Input: part model. Units: mm. Frame: model coordinates. A direction names the side the tool comes from. Round coordinates to 2 decimals unless told otherwise and drop trailing zeros. Write each loop counter-clockwise with the first axis right and the second up, starting at its lowest first coordinate (ties: lowest second). Pieces come first, ordered by that corner, then holes. Notation, with made-up numbers: (-21.5, 14.25) - (-10.5, 14.25) arc R32 ccw to (-10.5, 48.25) - close; hole circle Ø10 at (-5, 17.5). An arc over 180 degrees is marked (long way). Use one line per item in the form item = value.
Autodesk Inventor part; units mm, degrees
ref_plane "YZ Plane" through (0, 0, 0) normal (1, 0, 0) x (0, 1, 0)
ref_plane "XZ Plane" through (0, 0, 0) normal (0, 1, 0) x (-1, 0, 0)
ref_plane "XY Plane" through (0, 0, 0) normal (0, 0, 1) x (1, 0, 0)
sketch "Sketch1" plane through (0, 0, 0) normal (0, 0, 1) x (1, 0, 0)
  circle A0 centre (0, 0) radius 6
  dimension "d0" = 12
extrude "Extrusion1" add sketch "Sketch1" along normal blind 15
sketch "Sketch2" plane through (0, 0, 0) normal (0, 0, -1) x (-1, 0, 0)
  circle A0 centre (0, 0) radius 6
  circle A1 centre (0, 0) radius 4.699
  dimension "d3" = 9.398
extrude "Extrusion2" cut sketch "Sketch2" against normal blind 7 contours A1
sketch "Sketch3" plane through (0, 0, 15) normal (0, 0, 1) x (1, 0, 0)
  circle A0 centre (0, 0) radius 6
  circle A1 centre (0, 0) radius 3
  dimension "d6" = 6
extrude "Extrusion3" cut sketch "Sketch3" against normal blind 2.5 contours A1
sketch "Sketch4" plane through (0, 0, 15) normal (0, 0, 1) x (1, 0, 0)
  circle A0 centre (0, 0) radius 3
  circle A1 centre (0, 0) radius 6
extrude "Extrusion4" add sketch "Sketch4" along normal blind 15
sketch "Sketch5" plane through (0, 0, 12.5) normal (0, 0, 1) x (1, 0, 0)
  circle A0 centre (0, 0) radius 3
extrude "Extrusion5" add sketch "Sketch5" along normal blind 15
sketch "Sketch6" plane through (0, 0, 30) normal (0, 0, 1) x (1, 0, 0)
  circle A0 centre (0, 0) radius 3
  circle A1 centre (0, 0) radius 6
extrude "Extrusion6" cut sketch "Sketch6" against normal blind 17.5
sketch "Sketch7" plane through (0, 0, 27.5) normal (0, 0, 1) x (1, 0, 0)
  circle A0 centre (0, 0) radius 3
extrude "Extrusion7" cut sketch "Sketch7" against normal blind 17.5
properties part number "Shaft Cap" material "ABS Plastic"
(1) Draft query along Y for faces 1 (the face through (-6, 0, 6)), 2 (the face through (-3, -1, 12.5)), 3 (the face through (0, 0, 7)). Return one class per face: released by +Y, released by -Y, zero draft, split by the parting line, or undercut.
Derived:
face_1 = split by the parting line
face_2 = zero draft
face_3 = undercut
(2) First-contact query: pin 1 Ø6 at (y, z) = (-3.5, 3) entering from +X; pin 2 Ø1.5 at (x, y) = (-2, 0.5) entering from -Z; pin 3 Ø6 at (y, z) = (-3.5, 9.5) entering from -X. Flat tips, straight axial feed; report the tip coordinate or a pass-through.
Derived:
pin_1 = 5.98
pin_2 = 7
pin_3 = -5.98
(3) Access query for faces 4 (the face through (0.61, 4.66, 3.45)), 5 (the face through (0, 0, 10)), 6 (the face through (-4, -3, 0)). Directions: +Z, -Z, +X, -X, +Y, -Y. A direction counts if a zero-diameter tool reaches every point of the face in a straight line with its end or side. Return the directions, or none.
Derived:
face_4 = -Z
face_5 = +Z
face_6 = -Z, +X, -X, +Y, -Y
(4) Cut plane D-D on y = 4.5. Output: boundary loops of the cut face in (x, z).
Derived:
outline = (-3.97, 0) - (-1.35, 0) - (-1.35, 7) - (1.35, 7) - (1.35, 0) - (3.97, 0) - (3.97, 12.5) - (-3.97, 12.5) - close
(5) Cut plane A-A on x = 0. Output: boundary loops of the cut face in (y, z), then the cut area to 3 significant figures.
Derived:
outline = (-6, 0) - (-4.7, 0) - (-4.7, 7) - (4.7, 7) - (4.7, 0) - (6, 0) - (6, 12.5) - (3, 12.5) - (3, 10) - (-3, 10) - (-3, 12.5) - (-6, 12.5) - close
area = 69.2 mm^2
(6) Cut plane C-C on z = 11. Output: boundary loops of the cut face in (x, y).
Derived:
outline = circle Ø12 at (0, 0); hole circle Ø6 at (0, 0)
(7) Material intervals for L1, parallel to Y at x = 0, z = 2.25; L2, parallel to Y at x = 0, z = 11.6; L3, parallel to X at y = -0.5, z = 4.5, sorted ascending.
Derived:
L1 = -6 to -4.7, 4.7 to 6
L2 = -6 to -3, 3 to 6
L3 = -5.98 to -4.67, 4.67 to 5.98
